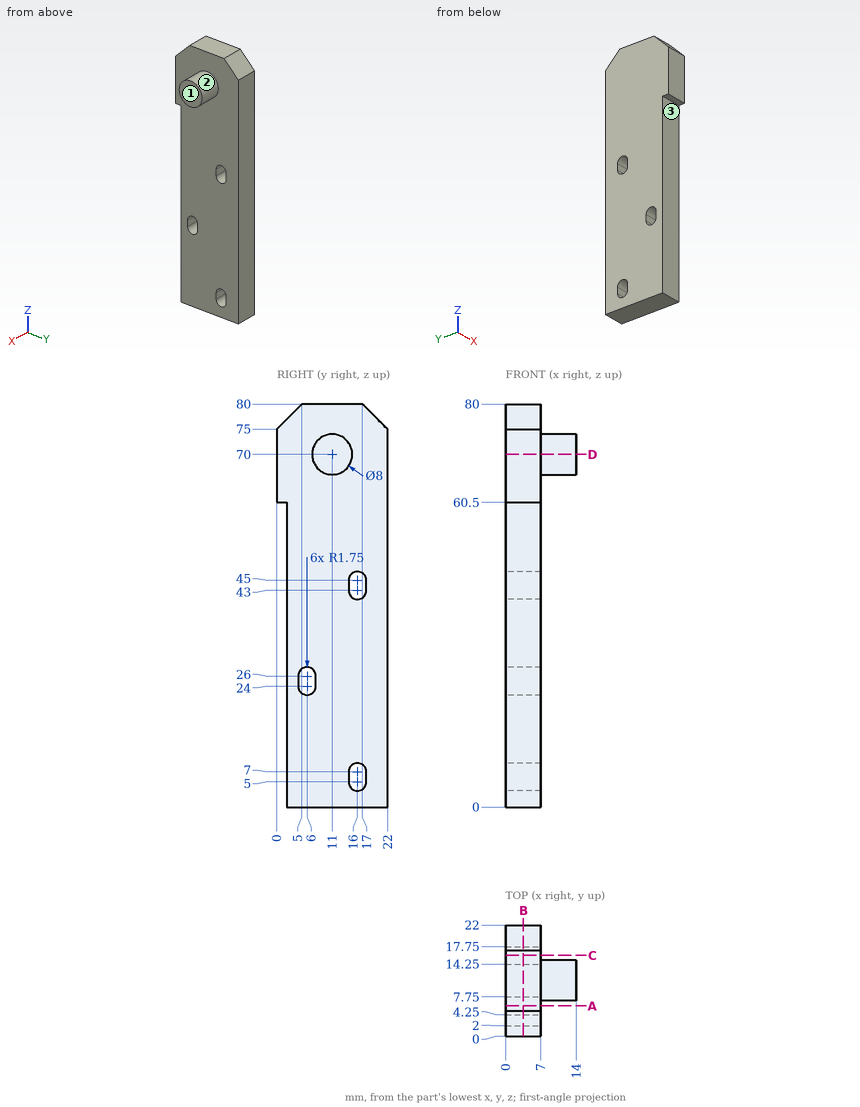
Geometry: see drawing. Coordinates: mm, zero at the bounding-box minimum. A direction names the side the tool comes from. Give positions to 0.01 mm unless a question says otherwise; leave off trailing zeros. Loops run counter-clockwise (first coordinate to the right, second up) from the corner with the lowest first, then second, coordinate; pieces in that order, holes last. Notation, with made-up numbers: (24, -37.5) -> (30, -37.5) arc R19 cw to (30, -11.5) -> close; hole circle Ø10 at (59, 62.5). An arc over 180 degrees is marked (long way). Answer as a JSON object with one key per item and string values. Group by question number.
Item 1: Cut plane D-D, the plane z = 70. Return the cut outline in (x, y), and give its area (3 significant figures).
Item 2: Cut plane A-A, the plane y = 6. Return the cut outline in (x, z).
Item 3: Cut plane B-B, the plane x = 3.5. Return the cut outline in (y, z), and give its area (3 significant figures).
Item 4: Cut plane C-C, the plane y = 16. Return the cut outline in (x, z).
Item 5: Line query: probe 1 along X at (y, z) = (20.25, 11); probe 2 along Y at (x, z) = (5.5, 30); probe 3 along Y at (x, z) = (6.5, 42.5). Output: solid intervals per line, ascending.
Item 6: Reachability of the marked faces 1, 2 and 3 from +Z, -Z, +X, -X, +Y, -Y: full face, straight path, thin tool, end or side. Return the list, or none.
Item 7: Pin query (flat end, axial travel): P1, Ø6, axis at y = 7.5, z = 41, coming from the +X side; P2, Ø2, axis at x = 2, y = 1.5, coming from the -Z side; P3, Ø0.6, axis at x = 4.5, z = 25.5, coming from the -Y side; P4, Ø1, axis at x = 8.5, y = 11.5, coming from the +Z side. Return the tip coordinate at first contact, or that it passes through.
Checks:
{
 "1": {"outline": "(0, 0) -> (7, 0) -> (7, 7) -> (14, 7) -> (14, 15) -> (7, 15) -> (7, 22) -> (0, 22) -> close", "area": "210 mm²"},
 "2": {"outline": "(0, 0) -> (7, 0) -> (7, 22.25) -> (0, 22.25) -> close; (0, 27.75) -> (7, 27.75) -> (7, 80) -> (0, 80) -> close"},
 "3": {"outline": "(0, 60.5) -> (2, 60.5) -> (2, 0) -> (22, 0) -> (22, 75) -> (17, 80) -> (5, 80) -> (0, 75) -> close; hole (4.25, 24) arc R1.75 ccw to (7.75, 24) -> (7.75, 26) arc R1.75 ccw to (4.25, 26) -> close; hole (14.25, 5) arc R1.75 ccw to (17.75, 5) -> (17.75, 7) arc R1.75 ccw to (14.25, 7) -> close; hole (14.25, 43) arc R1.75 ccw to (17.75, 43) -> (17.75, 45) arc R1.75 ccw to (14.25, 45) -> close", "area": "1,560 mm²"},
 "4": {"outline": "(0, 0) -> (7, 0) -> (7, 3.25) -> (0, 3.25) -> close; (0, 8.75) -> (7, 8.75) -> (7, 41.25) -> (0, 41.25) -> close; (0, 46.75) -> (7, 46.75) -> (7, 80) -> (0, 80) -> close"},
 "5": {"probe 1": "x = 0 to 7", "probe 2": "y = 2 to 22", "probe 3": "y = 2 to 14.32, 17.68 to 22"},
 "6": {"face 1": "+Z, -Z, +X, +Y, -Y", "face 2": "+X", "face 3": "-Z, +X, -X, -Y"},
 "7": {"P1": "stops at x = 7", "P2": "stops at z = 0", "P3": "stops at y = 2", "P4": "stops at z = 74"}
}
